from build123d import *

# Parameters (mm, degrees)
SKETCH1_W           = 40
SKETCH1_H           = 40
BOSS_EXTRUDE1_DEPTH = 25
CHAMFER1_SIZE       = 5
CHAMFER2_SIZE       = 5
CHAMFER3_SIZE       = 5
CHAMFER4_SIZE       = 5
SHELL1_T            = -2
SKETCH7_W           = 10
SKETCH7_H           = 24.34314575
BOSS_EXTRUDE6_DEPTH = 10
CUT_EXTRUDE2_DEPTH  = 24.343146
SKETCH11_W          = 10
SKETCH11_H          = 24.34314575
BOSS_EXTRUDE8_DEPTH = 2.828427
CUT_EXTRUDE4_DEPTH  = 58.096498152


with BuildPart() as part:
    # Sketch1 → Boss-Extrude1 (new body)
    with BuildSketch(Plane.XY):
        with Locations((20, -20)):
            Rectangle(SKETCH1_W, SKETCH1_H)
    extrude(amount=BOSS_EXTRUDE1_DEPTH)

    # Chamfer1
    chamfer1_edges = [part.edges().sort_by_distance(p)[0] for p in [
        (0, -20, 0),
    ]]
    chamfer(chamfer1_edges, length=CHAMFER1_SIZE)

    # Chamfer2
    chamfer2_edges = [part.edges().sort_by_distance(p)[0] for p in [
        (40, -20, 0),
    ]]
    chamfer(chamfer2_edges, length=CHAMFER2_SIZE)

    # Chamfer3
    chamfer3_edges = [part.edges().sort_by_distance(p)[0] for p in [
        (20, -40, 0),
    ]]
    chamfer(chamfer3_edges, length=CHAMFER3_SIZE)

    # Chamfer4
    chamfer4_edges = [part.edges().sort_by_distance(p)[0] for p in [
        (20, 0, 0),
    ]]
    chamfer(chamfer4_edges, length=CHAMFER4_SIZE)

    # Shell1
    shell1_openings = [part.faces().sort_by_distance(p)[0] for p in [
        (20, -20, 25),
        (20, -20, 0),
    ]]
    offset(amount=SHELL1_T, openings=shell1_openings, kind=Kind.INTERSECTION)



with BuildPart() as body_2:
    # Sketch7 → Boss-Extrude6 (new body)
    with BuildSketch(Plane(origin=(0, 0, 0), x_dir=(-1, 0, 0), z_dir=(0, 0, -1))):
        with Locations((-12.828427125, -20)):
            Rectangle(SKETCH7_W, SKETCH7_H)
    extrude(amount=BOSS_EXTRUDE6_DEPTH)

    # Sketch8 → Cut-Extrude2 (cut)
    with BuildSketch(Plane(origin=(0, -7.828427125, 0), x_dir=(1, 0, 0), z_dir=(0, 1, 0))):
        Polygon((7.828427125, 0), (17.828427125, 0), (17.828427125, 10), align=None)
    extrude(amount=-CUT_EXTRUDE2_DEPTH, mode=Mode.SUBTRACT)


with BuildPart() as part_1:
    add(part.part)

    add(body_2.part)  # Boss-Extrude8 merges body 2
    # Sketch11 → Boss-Extrude8 (add)
    with BuildSketch(Plane.ZY.offset(-7.828427125)):
        with Locations((-5, -20)):
            Rectangle(SKETCH11_W, SKETCH11_H)
    extrude(amount=BOSS_EXTRUDE8_DEPTH)

    # Sketch13 → Cut-Extrude4 (cut, through all)
    with BuildSketch(Plane(origin=(0, -7.828427125, 0), x_dir=(1, 0, 0), z_dir=(0, 1, 0))):
        Polygon((5, 0), (15, 10), (5, 10), align=None)
    extrude(amount=-CUT_EXTRUDE4_DEPTH, mode=Mode.SUBTRACT)


solid = part_1.part
The listing builds one solid part. Answer for the finished solid, in the listing's coordinates (mm). A direction names the side the tool comes from. Round coordinates to 2 decimals unless told otherwise and drop trailing zeros. Write each loop counter-clockwise with the first axis right and the second up, starting at its lowest first coordinate (ties: lowest second). Pieces come first, ordered by that corner, then holes. Notation, with made-up numbers: (52, -21.5) - (88, -21.5) arc R24 ccw to (88, 10.5) - close; hole circle Ø9 at (59, -26). An arc over 180 degrees is marked (long way). Use a Markdown table: item, result. Add a question column.
1. Consider line 1 (Y direction, x = 7.5, z = 10); line 2 (X direction, y = -14, z = 17); line 3 (X direction, y = -13, z = 3.5). Determine where each line is inside the solid, lowest interval first.
2. The part is cut by section C-C (x = 22.5). Write down the section's boundary in (y, z).
3. The part is cut by section A-A (y = -21). Write down the section's boundary in (x, z).
4. The part is cut by section B-B (z = 10). Write down the section's boundary in (x, y).
5. The part is cut by section D-D (x = 12.5). Write down the section's boundary in (y, z).
6. Flat-ended cylindrical pins translate along their axes: P1, Ø5, axis at x = 14.5, z = -4.5, coming from the -Y side; P2, Ø1, axis at x = 22, y = -32.5, coming from the +Z side; P3, Ø8, axis at x = 9.5, z = -7.5, coming from the +Y side. Find the tip coordinate at first contact, or state that the pin passes through.
7. A tool of negligible diameter and unlimited length cuts with its end or side. For faces 1 (the face through (2, -20, 15)), 2 (the face through (40, -20, 15)), from which of +Z, -Z, +X, -X, +Y, -Y can it reach the whole face along a straight path? Write none if from no direction.
8. For a pull along Y with two mould halves and no side action, classify faces 3 (the face through (6, -20, -1)), 4 (the face through (10.03, -19.75, -2.2)), 5 (the face through (38, -20, 15)), 6 (the face through (11, -32.172, -5)) as +Y half, -Y half, draft (parallel to the pull), parting line (faces both ways), or undercut.
Reported:
| question | item | result |
|---|---|---|
| 1 | line 1 | -40 to -38, -2 to 0 |
| 1 | line 2 | 0 to 2, 38 to 40 |
| 1 | line 3 | 1.5 to 4.33, 35.67 to 38.5 |
| 2 | outline | (-40, 5) - (-35, 0) - (-32.17, 0) - (-38, 5.83) - (-38, 25) - (-40, 25) - close; (-7.83, 0) - (-5, 0) - (0, 5) - (0, 25) - (-2, 25) - (-2, 5.83) - close |
| 3 | outline | (0, 5) - (15, -10) - (17.83, -10) - (2, 5.83) - (2, 25) - (0, 25) - close; (32.17, 0) - (35, 0) - (40, 5) - (40, 25) - (38, 25) - (38, 5.83) - close |
| 4 | outline | (0, -40) - (40, -40) - (40, 0) - (0, 0) - close; hole (2, -38) - (38, -38) - (38, -2) - (2, -2) - close |
| 5 | outline | (-40, 5) - (-35, 0) - (-32.17, 0) - (-38, 5.83) - (-38, 25) - (-40, 25) - close; (-32.17, -7.5) - (-7.83, -7.5) - (-7.83, -4.67) - (-32.17, -4.67) - close; (-7.83, 0) - (-5, 0) - (0, 5) - (0, 25) - (-2, 25) - (-2, 5.83) - close |
| 6 | P1 | y = -32.17 |
| 6 | P2 | z = 0.83 |
| 6 | P3 | y = -7.83 |
| 7 | face 1 | +Z |
| 7 | face 2 | +Z, -Z, +X, +Y, -Y |
| 8 | face 3 | draft |
| 8 | face 4 | undercut |
| 8 | face 5 | undercut |
| 8 | face 6 | -Y half |
